Here's how the part is built. I have some questions about the finished solid (model axes, mm). A direction names the side the tool comes from. Give positions to 0.01 mm unless a question says otherwise; leave off trailing zeros. Write each loop counter-clockwise with the first axis right and the second up, starting at its lowest first coordinate (ties: lowest second). Pieces come first, ordered by that corner, then holes. Notation, with made-up numbers: (-25.5, 16.5) - (10.5, 16.5) arc R27 cw to (10.5, 36.5) - close; hole circle Ø2 at (83, -31). An arc over 180 degrees is marked (long way). Use a Markdown table: item, result.
```python
from build123d import *

# Parameters (mm, degrees)
SKETCH1_R           = 5
SKETCH1_R_2         = 0.6
BOSS_EXTRUDE1_DEPTH = 7
SKETCH2_W           = 40
SKETCH2_H           = 5
BOSS_EXTRUDE2_DEPTH = 14
SKETCH3_R           = 1.5
CUT_EXTRUDE1_DEPTH  = 6


with BuildPart() as part:
    # Sketch1 → Boss-Extrude1 (new body)
    with BuildSketch(Plane.XY):
        with BuildLine():
            Line((20, 0), (20, -75))
            Line((20, -75), (-20, -75))
            Line((-20, -75), (-20, 0))
            ThreePointArc((-20, 0), (0, 20), (20, 0))
        make_face()
        Circle(SKETCH1_R, mode=Mode.SUBTRACT)
        with Locations((0, 7.25)):
            Circle(SKETCH1_R_2, mode=Mode.SUBTRACT)
        with Locations((-7.25, 0)):
            Circle(SKETCH1_R_2, mode=Mode.SUBTRACT)
        with Locations((0, -7.25)):
            Circle(SKETCH1_R_2, mode=Mode.SUBTRACT)
        with Locations((7.25, 0)):
            Circle(SKETCH1_R_2, mode=Mode.SUBTRACT)
    extrude(amount=BOSS_EXTRUDE1_DEPTH)

    # Sketch2 → Boss-Extrude2 (add)
    with BuildSketch(Plane.XY.offset(7)):
        with Locations((0, -72.5)):
            Rectangle(SKETCH2_W, SKETCH2_H)
    extrude(amount=BOSS_EXTRUDE2_DEPTH)

    # Sketch3 → Cut-Extrude1 (cut, through all)
    with BuildSketch(Plane(origin=(0, -70, 0), x_dir=(1, 0, 0), z_dir=(0, 1, 0))):
        with Locations((-10, -14)):
            Circle(SKETCH3_R)
        with Locations((10, -14)):
            Circle(SKETCH3_R)
    extrude(amount=-CUT_EXTRUDE1_DEPTH, mode=Mode.SUBTRACT)


solid = part.part
```
Item 1: Will these pins go through, and if not, where does the flat tip stop? pin 1 Ø1.6 at (x, y) = (0, -7.25) entering from +Z; pin 2 Ø6 at (x, z) = (-9, 2.5) entering from +Y; pin 3 Ø0.7 at (x, y) = (7.25, 0) entering from -Z; pin 4 Ø11 at (x, z) = (-1.5, 14.5) entering from +Y.
Values:
| item | result |
|---|---|
| pin 1 | stops at z = 7 |
| pin 2 | stops at y = 19.08 |
| pin 3 | passes through |
| pin 4 | stops at y = -70 |
Item 2: I need wall thicknesses on line 1 along Y through (x, z) = (0, 3); line 2 along X through (y, z) = (-72.6, 14); line 3 along Z through (x, y) = (10, -71.8). Which ranges of each line are inside material? Lowest first, please. Write a range as [from, to].
Values:
| item | result |
|---|---|
| line 1 | y = [-75, -7.85], [-6.65, -5], [5, 6.65], [7.85, 20] |
| line 2 | x = [-20, -11.5], [-8.5, 8.5], [11.5, 20] |
| line 3 | z = [0, 12.5], [15.5, 21] |
Item 3: If we section it at A-A, the plane y = -4: Write out the boundary of the cut face in (x, z), plus the area to 3 significant figures.
Values:
| item | result |
|---|---|
| outline | (-20, 0) - (-3, 0) - (-3, 7) - (-20, 7) - close; (3, 0) - (20, 0) - (20, 7) - (3, 7) - close |
| area | 238 mm2 |
Item 4: If we section it at C-C, the plane x = 10: Write out the boundary of the cut face in (y, z).
Values:
| item | result |
|---|---|
| outline | (-75, 0) - (17.32, 0) - (17.32, 7) - (-70, 7) - (-70, 12.5) - (-75, 12.5) - close; (-75, 15.5) - (-70, 15.5) - (-70, 21) - (-75, 21) - close |
Item 5: If we section it at B-B, the plane z = 14: Write out the boundary of the cut face in (x, y).
Values:
| item | result |
|---|---|
| outline | (-20, -75) - (-11.5, -75) - (-11.5, -70) - (-20, -70) - close; (-8.5, -75) - (8.5, -75) - (8.5, -70) - (-8.5, -70) - close; (11.5, -75) - (20, -75) - (20, -70) - (11.5, -70) - close |
Item 6: Thinking about a two-plate mould opening in X: for faces 1 (the flat face through (0, -72, 21)), 2 (the cylindrical face through (0, 20, 3)), 3 (the cylindrical face through (-1.08, -4.88, 3.45)), which applies, +X half, -X half, draft (parallel to the pull), parting line (faces both ways), or undercut?
Values:
| item | result |
|---|---|
| face 1 | draft |
| face 2 | parting line |
| face 3 | undercut |
Item 7: If we section it at D-D, the plane z = 3.5: Write out the boundary of the cut face in (x, y).
Values:
| item | result |
|---|---|
| outline | (-20, -75) - (20, -75) - (20, 0) arc R20 ccw to (-20, 0) - close; hole circle Ø1.2 at (-7.25, 0); hole circle Ø10 at (0, 0); hole circle Ø1.2 at (0, -7.25); hole circle Ø1.2 at (0, 7.25); hole circle Ø1.2 at (7.25, 0) |
Item 8: For faces 4 (the flat face through (0, -24, 7)), 5 (the flat face through (-20, -46, 6)), which set-ups out of +Z, -Z, +X, -X, +Y, -Y let a thin tool reach every point of the face, with its end or its side?
Values:
| item | result |
|---|---|
| face 4 | +Z, +X, -X, +Y |
| face 5 | +Z, -Z, -X, +Y, -Y |
